Geometry check sheet. Reference: the model listing, model coordinates, mm. Face numbers are marked on the shaded views. Round coordinates to 2 decimals unless told otherwise and drop trailing zeros. Order: outer loops, then holes, each group sorted by start corner. A loop starts at its lowest first (then second) coordinate and runs counter-clockwise, first axis right, second up. Notation, with made-up numbers: (63.25, 69) - (75.25, 69) arc R23 cw to (75.25, 92) - close; hole circle Ø3 at (65.25, 65). An arc over 180 degrees is marked (long way). Use a Markdown table: item, result. Add a question column.
(1) Section check D-D on z = -2. Record the boundary of the cut face in (x, y).
(2) Mould release check, pull along X, two halves, no side actions. Record for the marked faces 1, 2 and 3: released by +X, released by -X, zero draft, split by the parting line, or undercut.
(3) Section check B-B on z = 6. Record the boundary of the cut face in (x, y), then the cut area to 3 significant figures.
(4) Thickness scan on line 1 along Y through (x, z) = (0, 4.15); line 2 along X through (y, z) = (-1, -0.75); line 3 along Y through (x, z) = (41, -0.75). Record the ranges inside material, lowest first. Write a range as [from, to].
(5) Gauge pin test, flat ends, axial feed: P1, Ø3, axis at x = 20.5, y = 7, coming from the +Z side; P2, Ø1.6, axis at x = 22, z = 2.5, coming from the +Y side; P3, Ø1.6, axis at x = 26.5, z = 2, coming from the -Y side; P4, Ø4, axis at x = 0, y = 0, coming from the -Z side. Record the tip position at first contact, or that the pin passes through.
(6) Section check A-A on y = 0. Record the boundary of the cut face in (x, z).
(7) Section check C-C on x = 44.5. Record the boundary of the cut face in (y, z), then the cut area to 3 significant figures.
```python
from build123d import *

# Parameters (mm, degrees)
BOSS_EXTRU_1_DEPTH      = 3
BOSS_EXTRU_1_DEPTH_BACK = 3
ESQUISSE2_R             = 1.55
ENL_V_MAT_EXTRU_1_DEPTH = 6
SKETCH1_R               = 5
SKETCH1_R_2             = 1.55
BOSS_EXTRUDE1_DEPTH     = 5
BOSS_EXTRUDE3_DEPTH     = 4
FILLET1_R               = 2


with BuildPart() as part:
    # Esquisse1 → Boss.-Extru.1 (new, two sides: drawn at the far end of the back side and taken through both)
    with BuildSketch(Plane.XY.offset(-BOSS_EXTRU_1_DEPTH_BACK)):
        with BuildLine():
            Line((2.370532565, 4.402337488), (38.670532565, 4.402337488))
            ThreePointArc((38.670532565, 4.402337488), (46.041065131, 0), (38.670532565, -4.402337488))
            Line((38.670532565, -4.402337488), (2.370532565, -4.402337488))
            ThreePointArc((2.370532565, -4.402337488), (-5, 0), (2.370532565, 4.402337488))
        make_face()
    extrude(amount=BOSS_EXTRU_1_DEPTH + BOSS_EXTRU_1_DEPTH_BACK)

    # Esquisse2 → Enlèv. mat.-Extru.1 (cut)
    with BuildSketch(Plane.XY.offset(3)):
        Circle(ESQUISSE2_R)
        with Locations((41.041065131, 0)):
            Circle(ESQUISSE2_R)
    extrude(amount=-ENL_V_MAT_EXTRU_1_DEPTH, mode=Mode.SUBTRACT)

    # Sketch1 → Boss-Extrude1 (add)
    # profile 1 of 2: a face of its own
    with BuildSketch(Plane.XY.offset(3)):
        Circle(SKETCH1_R)
        Circle(SKETCH1_R_2, mode=Mode.SUBTRACT)
    # profile 2 of 2: a face of its own
    with BuildSketch(Plane.XY.offset(3)):
        with Locations((41.041065131, 0)):
            Circle(SKETCH1_R)
        with Locations((41.041065131, 0)):
            Circle(SKETCH1_R_2, mode=Mode.SUBTRACT)
    extrude(amount=BOSS_EXTRUDE1_DEPTH)

    # Sketch3 → Boss-Extrude3 (add)
    with BuildSketch(Plane(origin=(0, 0, -3), x_dir=(-1, 0, 0), z_dir=(0, 0, -1))):
        with BuildLine():
            Line((-0.036278369, 20.080410503), (7.604339365, 20.080410503))
            Line((7.604339365, 20.080410503), (7.604339365, -0.784525769))
            ThreePointArc((7.604339365, -0.784525769), (4.435345697, -6.226489092), (-1.743406195, -7.443251487))
            ThreePointArc((-1.743406195, -7.443251487), (-11.242367754, -7.816197838), (-20.642918726, -6.402337488))
            ThreePointArc((-20.642918726, -6.402337488), (-29.656725646, -5.741977649), (-38.670532565, -6.402337488))
            ThreePointArc((-38.670532565, -6.402337488), (-47.868169198, 0), (-38.670532565, 6.402337488))
            ThreePointArc((-38.670532565, 6.402337488), (-30.098734584, 5.912843699), (-21.526936603, 6.402337488))
            ThreePointArc((-21.526936603, 6.402337488), (-8.31538788, 9.366509266), (-0.036278369, 20.080410503))
        make_face()
        with BuildLine():
            Line((-38.670532565, 4.402337488), (-2.370532565, 4.402337488))
            ThreePointArc((-2.370532565, 4.402337488), (5, 0), (-2.370532565, -4.402337488))
            Line((-2.370532565, -4.402337488), (-38.670532565, -4.402337488))
            ThreePointArc((-38.670532565, -4.402337488), (-46.041065131, 0), (-38.670532565, 4.402337488))
        make_face(mode=Mode.SUBTRACT)
    extrude(amount=-BOSS_EXTRUDE3_DEPTH)

    # Fillet1
    fillet1_edges = [part.edges().sort_by_distance(p)[0] for p in [
        (0.036278369, 20.080410503, -1),
        (-7.604339365, 20.080410503, -1),
    ]]
    fillet(fillet1_edges, radius=FILLET1_R)


solid = part.part
```
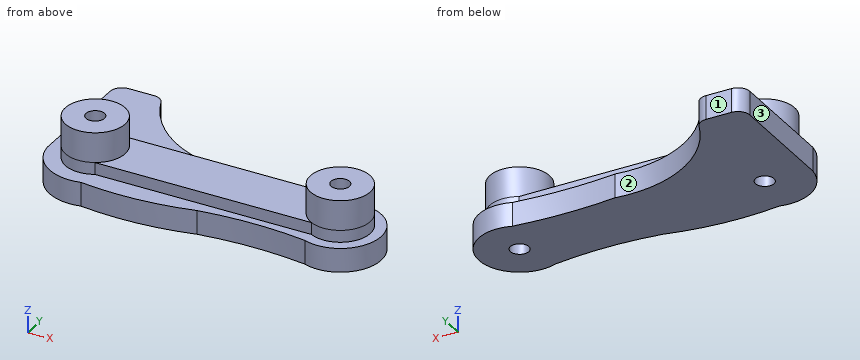
Check sheet entries:
| question | item | result |
|---|---|---|
| 1 | outline | (-7.6, -0.78) arc R7.64 ccw to (1.74, -7.44) arc R50.5 ccw to (20.64, -6.4) arc R61.85 cw to (38.67, -6.4) arc R6.83 ccw (long way) to (38.67, 6.4) arc R75.3 cw to (21.53, 6.4) arc R19.96 cw to (0.49, 18.82) arc R2 ccw to (-1.37, 20.08) - (-5.6, 20.08) arc R2 ccw to (-7.6, 18.08) - close; hole circle Ø3.1 at (0, 0); hole circle Ø3.1 at (41.04, 0) |
| 2 | face 1 | zero draft |
| 2 | face 2 | undercut |
| 2 | face 3 | released by -X |
| 3 | outline | circle Ø10 at (0, 0); circle Ø10 at (41.04, 0); hole circle Ø3.1 at (0, 0); hole circle Ø3.1 at (41.04, 0) |
| 3 | area | 142 mm2 |
| 4 | line 1 | y = [-5, -1.55], [1.55, 5] |
| 4 | line 2 | x = [-7.58, -1.18], [1.18, 39.86], [42.23, 47.79] |
| 4 | line 3 | y = [-6.83, -1.55], [1.55, 6.83] |
| 5 | P1 | stops at z = 1 |
| 5 | P2 | stops at y = 4.4 |
| 5 | P3 | stops at y = -4.4 |
| 5 | P4 | stops at z = -3 |
| 6 | outline | (-7.6, -3) - (-1.55, -3) - (-1.55, 8) - (-5, 8) - (-5, 1) - (-7.6, 1) - close; (1.55, -3) - (39.49, -3) - (39.49, 8) - (36.04, 8) - (36.04, 3) - (5, 3) - (5, 8) - (1.55, 8) - close; (42.59, -3) - (47.87, -3) - (47.87, 1) - (46.04, 1) - (46.04, 8) - (42.59, 8) - close |
| 7 | outline | (-5.89, -3) - (5.89, -3) - (5.89, 1) - (3.61, 1) - (3.61, 8) - (-3.61, 8) - (-3.61, 1) - (-5.89, 1) - close |
| 7 | area | 97.6 mm2 |
